Geometry: final body of the model. Coordinates: model frame, mm. A direction names the side the tool comes from. Give positions to 0.01 mm unless a question says otherwise; leave off trailing zeros. Order: outer loops, then holes, each group sorted by start corner. A loop starts at its lowest first (then second) coordinate and runs counter-clockwise, first axis right, second up. Notation, with made-up numbers: (-18.75, -3) -> (17.25, -3) arc R6 cw to (17.25, 1) -> close; hole circle Ø7 at (-1, 88.5). An arc over 180 degrees is marked (long way). One line per question, with ' | ' between items.
from build123d import *

# Parameters (mm, degrees)
F0_W      = 113.8684004545
F0_H      = 36.3644612953
F1_DEPTH  = 25.4
F2_DEPTH  = 50.8
F3_W      = 15.3176933527
F3_H      = 16.8904128104
F4_DEPTH  = 127
F5_W      = 19.7984315455
F5_H      = 18.0663006932
F6_DEPTH  = 127
F7_W      = 16.7733989656
F7_H      = 18.577855546
F9_DEPTH  = 127
F10_W     = 15.0831528008
F10_H     = 25.3941109404
F11_DEPTH = 25.4
F12_W     = 15.0831528008
F12_H     = 25.3941109404
F13_DEPTH = 101.6
F14_W     = 31.9914445281
F14_H     = 31.2603749335
F15_DEPTH = 2.54
F16_W     = 27.1054208279
F16_H     = 30.2256134719
F17_DEPTH = 2.54
F18_W     = 38.1215699017
F18_H     = 29.6914111823
F19_DEPTH = 1
F20_W     = 30.2939862013
F20_H     = 27.2640747398
F21_DEPTH = 2.54


with BuildPart() as f1:
    # F0 (on Top) → F1 (new body)
    with BuildSketch(Plane.XY):
        with Locations((-0.5311109126, -5.1947091706)):
            Rectangle(F0_W, F0_H)
    extrude(amount=F1_DEPTH)

    # F2 (add): a face of the model
    f2_faces = [f1.faces().sort_by_distance(p)[0] for p in [
        (-0.5311109126, -23.3769398183, 12.7),
    ]]
    extrude(f2_faces, amount=F2_DEPTH)

    # F3 (on face) → F4 (join)
    with BuildSketch(Plane(origin=(0, 0, 0), x_dir=(1, 0, 0), z_dir=(0, 0, -1))):
        with Locations((48.7442426383, 65.731733413)):
            Rectangle(F3_W, F3_H)
    extrude(amount=F4_DEPTH)

    # F5 (on face) → F6 (join)
    with BuildSketch(Plane(origin=(0, 0, 0), x_dir=(1, 0, 0), z_dir=(0, 0, -1))):
        with Locations((-47.5660953671, 65.1437894717)):
            Rectangle(F5_W, F5_H)
    extrude(amount=F6_DEPTH)

    # F7 (on face) → F9 (join)
    with BuildSketch(Plane(origin=(0, 0, 0), x_dir=(1, 0, 0), z_dir=(0, 0, -1))):
        with Locations((48.0163898319, -3.698593704)):
            Rectangle(F7_W, F7_H)
    extrude(amount=F9_DEPTH)

    # F10 (on face) → F11 (join)
    with BuildSketch(Plane(origin=(0, 0, 0), x_dir=(1, 0, 0), z_dir=(0, 0, -1))):
        with Locations((-48.6456360668, -1.0305386968)):
            Rectangle(F10_W, F10_H)
    extrude(amount=F11_DEPTH)

    # F12 (on face) → F13 (join)
    with BuildSketch(Plane(origin=(0, 0, -25.4), x_dir=(1, 0, 0), z_dir=(0, 0, -1))):
        with Locations((-48.6456360668, -1.0305386968)):
            Rectangle(F12_W, F12_H)
    extrude(amount=F13_DEPTH)

    # F14 (on face) → F15 (join)
    with BuildSketch(Plane(origin=(0, 0, -127), x_dir=(1, 0, 0), z_dir=(0, 0, -1))):
        with Locations((-48.9207692444, 0)):
            Rectangle(F14_W, F14_H)
    extrude(amount=F15_DEPTH)

    # F16 (on face) → F17 (join)
    with BuildSketch(Plane(origin=(0, 0, -127), x_dir=(1, 0, 0), z_dir=(0, 0, -1))):
        with Locations((-47.1377819777, 65.1437894717)):
            Rectangle(F16_W, F16_H)
    extrude(amount=F17_DEPTH)

    # F18 (on face) → F19 (join)
    with BuildSketch(Plane(origin=(0, 0, -127), x_dir=(1, 0, 0), z_dir=(0, 0, -1))):
        with Locations((48.0163898319, 0)):
            Rectangle(F18_W, F18_H)
    extrude(amount=F19_DEPTH)

    # F20 (on face) → F21 (join)
    with BuildSketch(Plane(origin=(0, 0, -127), x_dir=(1, 0, 0), z_dir=(0, 0, -1))):
        with Locations((48.7307161093, 65.731733413)):
            Rectangle(F20_W, F20_H)
    extrude(amount=F21_DEPTH)


solid = f1.part
1) Section D-D on x = 14. Return loops of the section in (y, z), plus the area to 3 significant figures.
Check result:
outline: (-74.18, 0) -> (12.99, 0) -> (12.99, 25.4) -> (-74.18, 25.4) -> close | area: 2,210 mm^2
2) Section B-B on x = -48. Return loops of the section in (y, z).
Check result:
outline: (-80.26, -129.54) -> (-50.03, -129.54) -> (-50.03, -127) -> (-56.11, -127) -> (-56.11, 0) -> (-11.67, 0) -> (-11.67, -127) -> (-15.63, -127) -> (-15.63, -129.54) -> (15.63, -129.54) -> (15.63, -127) -> (13.73, -127) -> (13.73, 0) -> (12.99, 0) -> (12.99, 25.4) -> (-74.18, 25.4) -> (-74.18, -127) -> (-80.26, -127) -> close
3) Material intervals for probe 1 along Y at (x, z) = (54, -10.5); probe 2 along Z at (x, y) = (53.5, -54); probe 3 along X at (y, z) = (-71.5, -115), sorted ascending. Write a range as from..to.
Check result:
probe 1: y = -74.18..-57.29, -5.59..12.99 | probe 2: z = -129.54..-127, 0..25.4 | probe 3: x = -57.47..-37.67, 41.09..56.4
4) Pull-direction query (Y, two-part tool) for faces 1 (the flat face through (-1, -30, 0)), 2 (the flat face through (-1, -30, 25.4)), 3 (the flat face through (-49, 13.728, -63)); classes: +Y half, -Y half, draft (parallel to the pull), parting line (faces both ways), or undercut.
Check result:
face 1: undercut | face 2: draft | face 3: +Y half
5) Section C-C on y = -25.5. Return loops of the section in (x, z), plus the area to 3 significant figures.
Check result:
outline: (-57.47, 0) -> (56.4, 0) -> (56.4, 25.4) -> (-57.47, 25.4) -> close | area: 2,890 mm^2
6) Contact query for flat-ended pins moving along their axis: pin 1 Ø16.5 at (x, z) = (-45.5, -88) entering from +Y; pin 2 Ø2 at (y, z) = (-61, -128) entering from -X; pin 3 Ø0.8 at (x, z) = (56, -128) entering from -Y. Output: stop coordinate, or through.
Check result:
pin 1: stops at y = 13.73 | pin 2: stops at x = -60.69 | pin 3: stops at y = -79.36
7) Set-up query: faces 4 (the flat face through (-39, -74.177, -33)), 5 (the flat face through (-37.667, -65, -63)), 6 (the flat face through (-48, -56.111, -63)). Return all of +Z, -Z, +X, -X, +Y, -Y with unobstructed straight access to the full face (end or side cutting, diameter ignored); none if empty.
Check result:
face 4: +Z, +X, -X, -Y | face 5: +Y, -Y | face 6: +X, -X
8) Section A-A on z = -63. Return loops of the section in (x, y).
Check result:
outline: (-57.47, -74.18) -> (-37.67, -74.18) -> (-37.67, -56.11) -> (-57.47, -56.11) -> close; (-56.19, -11.67) -> (-41.1, -11.67) -> (-41.1, 13.73) -> (-56.19, 13.73) -> close; (39.63, -5.59) -> (56.4, -5.59) -> (56.4, 12.99) -> (39.63, 12.99) -> close; (41.09, -74.18) -> (56.4, -74.18) -> (56.4, -57.29) -> (41.09, -57.29) -> close
